from build123d import *

# Parameters (mm, degrees)
BOSS_EXTRUDE1_DEPTH = 10
SKETCH2_R           = 3.5
BOSS_EXTRUDE2_DEPTH = 7
SKETCH5_OUTSIDE_W   = 12.934
SKETCH5_OUTSIDE_H   = 12.934
CUT_EXTRUDE1_DEPTH  = 6


with BuildPart() as part:
    # Sketch1 → Boss-Extrude1 (new body)
    with BuildSketch(Plane.XY):
        Polygon((3.4, 0), (1.7, 2.944486373), (-1.7, 2.944486373), (-3.4, 0), (-1.7, -2.944486373), (1.7, -2.944486373), align=None)
    extrude(amount=BOSS_EXTRUDE1_DEPTH)

    # Sketch2 → Boss-Extrude2 (add)
    with BuildSketch(Plane.XY.offset(10)):
        Circle(SKETCH2_R)
    extrude(amount=BOSS_EXTRUDE2_DEPTH)

    # Sketch5 outside → Cut-Extrude1 (cut)
    with BuildSketch(Plane.XY.offset(17)):
        Rectangle(SKETCH5_OUTSIDE_W, SKETCH5_OUTSIDE_H)
        with BuildLine():
            ThreePointArc((-1.225048855, -2.680805064), (-1.222210326, -2.658421079), (-1.220475879, -2.635924597))
            ThreePointArc((-1.220475879, -2.635924597), (-1.430570177, -2.226010646), (-1.890717348, -2.20518656))
            ThreePointArc((-1.890717348, -2.20518656), (-1.910460352, -2.216109645), (-1.929642373, -2.227990304))
            ThreePointArc((-1.929642373, -2.227990304), (-2.205665987, -2.368094557), (-2.505525497, -2.444922359))
            ThreePointArc((-2.505525497, -2.444922359), (-2.645696022, -2.292508653), (-2.776610031, -2.13207413))
            ThreePointArc((-2.776610031, -2.13207413), (-2.657889767, -1.846200494), (-2.479929318, -1.592925316))
            ThreePointArc((-2.479929318, -1.592925316), (-2.4654397, -1.575629335), (-2.451818074, -1.557641803))
            ThreePointArc((-2.451818074, -1.557641803), (-2.40694443, -1.09921469), (-2.782786513, -0.832922011))
            ThreePointArc((-2.782786513, -0.832922011), (-2.80530085, -0.831437221), (-2.827860963, -0.831061285))
            ThreePointArc((-2.827860963, -0.831061285), (-3.135812881, -0.79969485), (-3.429606999, -0.702210219))
            ThreePointArc((-3.429606999, -0.702210219), (-3.465124877, -0.498209743), (-3.488519299, -0.292466177))
            ThreePointArc((-3.488519299, -0.292466177), (-3.234090501, -0.116158991), (-2.947449745, 0.000696964))
            ThreePointArc((-2.947449745, 0.000696964), (-2.925909389, 0.00741359), (-2.904725354, 0.015181258))
            ThreePointArc((-2.904725354, 0.015181258), (-2.619130834, 0.376574163), (-2.791340622, 0.80378939))
            ThreePointArc((-2.791340622, 0.80378939), (-2.80947815, 0.817210645), (-2.828253678, 0.829723821))
            ThreePointArc((-2.828253678, 0.829723821), (-3.070361342, 1.022602322), (-3.264812511, 1.263448704))
            ThreePointArc((-3.264812511, 1.263448704), (-3.184401067, 1.454267239), (-3.092848337, 1.63999772))
            ThreePointArc((-3.092848337, 1.63999772), (-2.783490351, 1.65076217), (-2.479175704, 1.594097963))
            ThreePointArc((-2.479175704, 1.594097963), (-2.457423521, 1.588102753), (-2.435402858, 1.583184377))
            ThreePointArc((-2.435402858, 1.583184377), (-1.999761704, 1.73280338), (-1.913663807, 2.18530334))
            ThreePointArc((-1.913663807, 2.18530334), (-1.921665988, 2.206399906), (-1.930695833, 2.227077476))
            ThreePointArc((-1.930695833, 2.227077476), (-2.030091771, 2.520230481), (-2.063463119, 2.82797159))
            ThreePointArc((-2.063463119, 2.82797159), (-1.892652419, 2.945024649), (-1.715219882, 3.051773929))
            ThreePointArc((-1.715219882, 3.051773929), (-1.449151682, 2.893578006), (-1.223780893, 2.681384122))
            ThreePointArc((-1.223780893, 2.681384122), (-1.208723048, 2.664580512), (-1.192857163, 2.648537642))
            ThreePointArc((-1.192857163, 2.648537642), (-0.745482362, 2.538879767), (-0.428412254, 2.87299892))
            ThreePointArc((-0.428412254, 2.87299892), (-0.423738452, 2.895072786), (-0.420155704, 2.917349768))
            ThreePointArc((-0.420155704, 2.917349768), (-0.345282406, 3.217703271), (-0.206978766, 3.494633479))
            ThreePointArc((-0.206978766, 3.494633479), (-0.103534673, 3.499226191), (0, 3.500757541))
            ThreePointArc((0, 3.500757541), (0.103534673, 3.499226191), (0.206978766, 3.494633479))
            ThreePointArc((0.206978766, 3.494633479), (0.345282406, 3.217703271), (0.420155704, 2.917349768))
            ThreePointArc((0.420155704, 2.917349768), (0.423738452, 2.895072786), (0.428412254, 2.87299892))
            ThreePointArc((0.428412254, 2.87299892), (0.745482362, 2.538879767), (1.192857163, 2.648537642))
            ThreePointArc((1.192857163, 2.648537642), (1.208723048, 2.664580512), (1.223780893, 2.681384122))
            ThreePointArc((1.223780893, 2.681384122), (1.449151682, 2.893578006), (1.715219882, 3.051773929))
            ThreePointArc((1.715219882, 3.051773929), (1.892652419, 2.945024649), (2.063463119, 2.82797159))
            ThreePointArc((2.063463119, 2.82797159), (2.030091771, 2.520230481), (1.930695833, 2.227077476))
            ThreePointArc((1.930695833, 2.227077476), (1.921665988, 2.206399906), (1.913663807, 2.18530334))
            ThreePointArc((1.913663807, 2.18530334), (1.999761704, 1.73280338), (2.435402858, 1.583184377))
            ThreePointArc((2.435402858, 1.583184377), (2.457423521, 1.588102753), (2.479175704, 1.594097963))
            ThreePointArc((2.479175704, 1.594097963), (2.783490351, 1.65076217), (3.092848337, 1.63999772))
            ThreePointArc((3.092848337, 1.63999772), (3.184401067, 1.454267239), (3.264812511, 1.263448704))
            ThreePointArc((3.264812511, 1.263448704), (3.070361342, 1.022602322), (2.828253678, 0.829723821))
            ThreePointArc((2.828253678, 0.829723821), (2.80947815, 0.817210645), (2.791340622, 0.80378939))
            ThreePointArc((2.791340622, 0.80378939), (2.619130834, 0.376574163), (2.904725354, 0.015181258))
            ThreePointArc((2.904725354, 0.015181258), (2.925909389, 0.00741359), (2.947449745, 0.000696964))
            ThreePointArc((2.947449745, 0.000696964), (3.234090501, -0.116158991), (3.488519299, -0.292466177))
            ThreePointArc((3.488519299, -0.292466177), (3.465124877, -0.498209743), (3.429606999, -0.702210219))
            ThreePointArc((3.429606999, -0.702210219), (3.135812881, -0.79969485), (2.827860963, -0.831061285))
            ThreePointArc((2.827860963, -0.831061285), (2.80530085, -0.831437221), (2.782786513, -0.832922011))
            ThreePointArc((2.782786513, -0.832922011), (2.40694443, -1.09921469), (2.451818074, -1.557641803))
            ThreePointArc((2.451818074, -1.557641803), (2.4654397, -1.575629335), (2.479929318, -1.592925316))
            ThreePointArc((2.479929318, -1.592925316), (2.657889767, -1.846200494), (2.776610031, -2.13207413))
            ThreePointArc((2.776610031, -2.13207413), (2.645696022, -2.292508653), (2.505525497, -2.444922359))
            ThreePointArc((2.505525497, -2.444922359), (2.205665989, -2.368094556), (1.929642376, -2.227990303))
            ThreePointArc((1.929642376, -2.227990303), (1.910460355, -2.216109643), (1.890717351, -2.205186558))
            ThreePointArc((1.890717351, -2.205186558), (1.430570178, -2.226010644), (1.220475879, -2.635924598))
            ThreePointArc((1.220475879, -2.635924598), (1.222210326, -2.65842108), (1.225048855, -2.680805065))
            ThreePointArc((1.225048855, -2.680805065), (1.237827812, -2.990086385), (1.183146697, -3.294763611))
            ThreePointArc((1.183146697, -3.294763611), (0.986277373, -3.358952263), (0.785957353, -3.411388925))
            ThreePointArc((0.785957353, -3.411388925), (0.575235727, -3.184640974), (0.418775964, -2.917548145))
            ThreePointArc((0.418775964, -2.917548145), (0.409062191, -2.897182914), (0.398358784, -2.877319957))
            ThreePointArc((0.398358784, -2.877319957), (0, -2.646063949), (-0.398358784, -2.877319956))
            ThreePointArc((-0.398358784, -2.877319956), (-0.409062191, -2.897182914), (-0.418775964, -2.917548145))
            ThreePointArc((-0.418775964, -2.917548145), (-0.575235727, -3.184640974), (-0.785957353, -3.411388925))
            ThreePointArc((-0.785957353, -3.411388925), (-0.986277373, -3.358952263), (-1.183146697, -3.294763611))
            ThreePointArc((-1.183146697, -3.294763611), (-1.237827813, -2.990086384), (-1.225048855, -2.680805064))
        make_face(mode=Mode.SUBTRACT)
    extrude(amount=-CUT_EXTRUDE1_DEPTH, mode=Mode.SUBTRACT)


solid = part.part
Design review of the part built by this model. Coordinates are the model's own, in mm. A direction names the side the tool comes from. Round coordinates to 2 decimals unless told otherwise and drop trailing zeros. Write each loop counter-clockwise with the first axis right and the second up, starting at its lowest first coordinate (ties: lowest second). Pieces come first, ordered by that corner, then holes. Notation, with made-up numbers: (-30.75, -35.5) - (25.25, -35.5) arc R28 cw to (25.25, -16.5) - close; hole circle Ø3 at (63, 66.5). An arc over 180 degrees is marked (long way). Return JSON: item names as keys, results as strings. Group by question number.
Item 1: We need section D-D on x = -1. Write out the cut boundary in (y, z).
Item 2: We need section C-C on y = -0.5. Write out the cut boundary in (x, z), and give its area (3 significant figures).
Item 3: The part is to be moulded in two halves that separate along X. For faces 1 (the face through (0, -2.944, 5)), 2 (the face through (-2.562, -1.452, 4.93)), 3 (the face through (0, -3, 11)), 4 (the face through (-1.7, -2.6, 11)), say which applies: pulls with the +X half, pulls with the -X half, needs draft (parallel to the pull), parting line crosses it, or undercut.
Item 4: We need section A-A on x = 0. Write out the cut boundary in (y, z), and give its area (3 significant figures).
Item 5: We need section B-B on z = 5. Write out the cut boundary in (x, y).
Item 6: Insertion check: P1, Ø0.6, axis at x = 2, y = -3, coming from the +Z side; P2, Ø1, axis at x = -1, z = 7, coming from the +Y side; P3, Ø1.3, axis at x = -2.5, y = 2.5, coming from the +Z side; P4, Ø3, axis at y = -2.5, z = 7.5, coming from the -X side. Each pin has a flat end and moves straight along its axis. Give the tip position at first contact, or say it passes through.
Item 7: Machinability: for faces 5 (the face through (-2.54, 1.49, 4.93)), 6 (the face through (3, -1, 11)), 7 (the face through (2.54, -1.49, 4.93)), 8 (the face through (-3.2, 0.5, 11)), 9 (the face through (-3, 1, 10)), which of the approach directions +Z, -Z, +X, -X, +Y, -Y give a long, thin tool a straight path to every point of the face, cutting with its end or side? Answer none if there is none.
Item 8: For probe 1 along Z at (x, y) = (-2, -2.5); probe 2 along Z at (x, y) = (-2.25, -2.25); probe 3 along Y at (x, z) = (0.75, 5.5), list the stretches that pass through material, from the lowest coordinate up. Write a range as [from, to].
Model answer:
{
 "1": {"outline": "(-3.35, 10) - (-2.94, 10) - (-2.94, 0) - (2.94, 0) - (2.94, 10) - (3.35, 10) - (3.35, 11) - (2.54, 11) - (2.54, 17) - (-3.35, 17) - close"},
 "2": {"outline": "(-3.46, 10) - (-3.11, 10) - (-3.11, 0) - (3.11, 0) - (3.11, 10) - (3.46, 10) - (3.46, 17) - (-3.46, 17) - close", "area": "111 mm²"},
 "3": {"face 1": "needs draft", "face 2": "pulls with the -X half", "face 3": "undercut", "face 4": "undercut"},
 "4": {"outline": "(-3.5, 10) - (-2.94, 10) - (-2.94, 0) - (2.94, 0) - (2.94, 10) - (3.5, 10) - (3.5, 17) - (-2.65, 17) - (-2.65, 11) - (-3.5, 11) - close", "area": "103 mm²"},
 "5": {"outline": "(-3.4, 0) - (-1.7, -2.94) - (1.7, -2.94) - (3.4, 0) - (1.7, 2.94) - (-1.7, 2.94) - close"},
 "6": {"P1": "stops at z = 11", "P2": "stops at y = 2.94", "P3": "stops at z = 17", "P4": "stops at x = -2.82"},
 "7": {"face 5": "-Z, -X, +Y", "face 6": "+Z, +X", "face 7": "-Z, +X, -Y", "face 8": "+Z, -X", "face 9": "-Z"},
 "8": {"probe 1": "z = [10, 11]", "probe 2": "z = [10, 17]", "probe 3": "y = [-2.94, 2.94]"}
}
